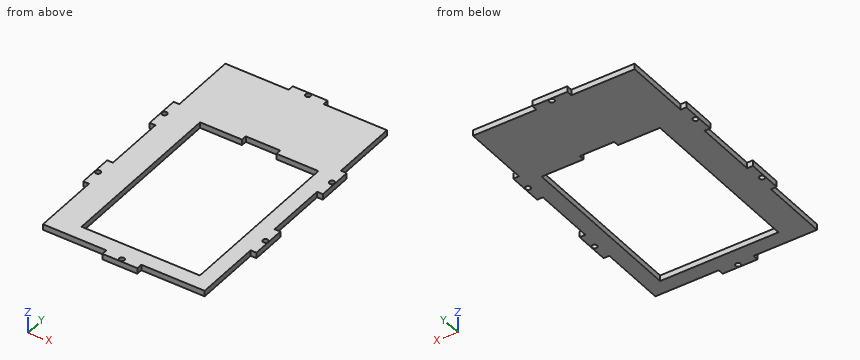
```python
from build123d import *

# Parameters (mm, degrees)
BOSS_EXTRUDE1_DEPTH     = 3.18
CUT_EXTRUDE1_DEPTH      = 87.179315674
SKETCH27_W              = 3.18
SKETCH27_H              = 19.3
BOSS_EXTRUDE9_DEPTH     = 3.18
SKETCH28_W              = 19.3
SKETCH28_H              = 3.18
BOSS_EXTRUDE10_DEPTH    = 3.18
SKETCH29_R              = 1.425
CUT_EXTRUDE14_DEPTH     = 91.550668965
SKETCH30_R              = 1.425
CUT_EXTRUDE15_DEPTH     = 91.550668965
MIRROR9_COPY_1_SKETCH_W = 3.18
MIRROR9_COPY_1_SKETCH_H = 19.3
MIRROR9_COPY_1_DEPTH    = 3.18
MIRROR9_COPY_2_SKETCH_R = 1.425
MIRROR9_COPY_2_DEPTH    = 91.550668965


with BuildPart() as part:
    # Sketch1 → Boss-Extrude1 (new body)
    with BuildSketch(Plane.XY):
        Polygon((-44.645, 73.645), (-14.881666667, 73.645), (14.881666667, 73.645), (44.645, 73.645), (44.645, -73.645), (-44.645, -73.645), align=None)
    extrude(amount=BOSS_EXTRUDE1_DEPTH)

    # Sketch3 → Cut-Extrude1 (cut, through all)
    with BuildSketch(Plane(origin=(0, 0, 0), x_dir=(-1, 0, 0), z_dir=(0, 0, -1))):
        Polygon((-13.10174207, 33.47325793), (-13.10174207, 30.47325793), (-36.27674207, 30.47325793), (-36.27674207, -65.27674207), (29.07325793, -65.27674207), (29.07325793, 30.47325793), (5.89825793, 30.47325793), (5.89825793, 33.47325793), align=None)
    extrude(amount=-CUT_EXTRUDE1_DEPTH, mode=Mode.SUBTRACT)

    # Sketch27 → Boss-Extrude9 (add)
    with BuildSketch(Plane.ZY.offset(44.645)):
        with Locations((1.59, -26.825)):
            Rectangle(SKETCH27_W, SKETCH27_H)
    boss_extrude9 = extrude(amount=BOSS_EXTRUDE9_DEPTH)

    # Sketch28 → Boss-Extrude10 (add)
    with BuildSketch(Plane.XZ.offset(73.645)):
        with Locations((0, 1.59)):
            Rectangle(SKETCH28_W, SKETCH28_H)
    boss_extrude10 = extrude(amount=BOSS_EXTRUDE10_DEPTH)

    # Sketch29 → Cut-Extrude14 (cut, through all)
    with BuildSketch(Plane.XY.offset(3.18)):
        with Locations((-46.235, -26.825)):
            Circle(SKETCH29_R)
    cut_extrude14 = extrude(amount=-CUT_EXTRUDE14_DEPTH, mode=Mode.SUBTRACT)

    # Sketch30 → Cut-Extrude15 (cut, through all)
    with BuildSketch(Plane.XY.offset(3.18)):
        with Locations((0, -75.235)):
            Circle(SKETCH30_R)
    cut_extrude15 = extrude(amount=-CUT_EXTRUDE15_DEPTH, mode=Mode.SUBTRACT)

    # Mirror8: Boss-Extrude9, Cut-Extrude14 across plane
    add(boss_extrude9.mirror(Plane(origin=(0, 0, 0), x_dir=(0, 0, 1), z_dir=(1, 0, 0))))
    add(cut_extrude14.mirror(Plane(origin=(0, 0, 0), x_dir=(0, 0, 1), z_dir=(1, 0, 0))), mode=Mode.SUBTRACT)

    # Mirror9: Boss-Extrude9, Boss-Extrude10, Cut-Extrude14, Cut-Extrude15 across plane
    add(boss_extrude9.mirror(Plane.ZX))
    add(boss_extrude10.mirror(Plane.ZX))
    add(cut_extrude14.mirror(Plane.ZX), mode=Mode.SUBTRACT)
    add(cut_extrude15.mirror(Plane.ZX), mode=Mode.SUBTRACT)

    # Mirror9 copy 1 sketch → Mirror9 copy 1 (add)
    with BuildSketch(Plane(origin=(44.645, 0, 0), x_dir=(0, 0, 1), z_dir=(1, 0, 0))):
        with Locations((1.59, -26.825)):
            Rectangle(MIRROR9_COPY_1_SKETCH_W, MIRROR9_COPY_1_SKETCH_H)
    extrude(amount=MIRROR9_COPY_1_DEPTH)

    # Mirror9 copy 2 sketch → Mirror9 copy 2 (cut, through all)
    with BuildSketch(Plane(origin=(0, 0, 3.18), x_dir=(-1, 0, 0), z_dir=(0, 0, 1))):
        with Locations((-46.235, -26.825)):
            Circle(MIRROR9_COPY_2_SKETCH_R)
    extrude(amount=-MIRROR9_COPY_2_DEPTH, mode=Mode.SUBTRACT)


solid = part.part
```
Geometry check sheet. Reference: the model listing, model coordinates, mm. Round coordinates to 2 decimals unless told otherwise and drop trailing zeros. Order: outer loops, then holes, each group sorted by start corner. A loop starts at its lowest first (then second) coordinate and runs counter-clockwise, first axis right, second up. Notation, with made-up numbers: (62.5, 19.25) - (110.5, 19.25) arc R37 ccw to (110.5, 57.25) - close; hole circle Ø10 at (21, 55). An arc over 180 degrees is marked (long way). Use a Markdown table: item, result. Add a question column.
(1) Sectioned sample at B-B, the plane x = 30.5. Enter the section's corners in (y, z) (3 decimals), and give its area (3 significant figures).
(2) Sectioned sample at D-D, the plane z = 0.7. Count the separate pieces of the cut face and the enclosed holes in it, and give its area (3 significant figures).
(3) Material ranges on line 1 along Y through (x, z) = (0, 0.9) (3 decimals); line 2 along X through (y, z) = (-58, 2.75) (3 decimals); line 3 along Y through (x, z) = (9, 3.05) (3 decimals), recorded low to high. Write a range as [from, to].
(4) Sectioned sample at C-C, the plane x = -35.5. Enter the section's corners in (y, z) (3 decimals), and give its area (3 significant figures).
(5) Depth check by flat-ended pin: pin 1 (1 mm diameter, centred on y = 76, z = 1, fed in from +X); pin 2 (1 mm diameter, centred on x = 46.5, z = 2.5, fed in from -Y) (3 decimals); pin 3 (1.6 mm diameter, centred on y = -11.5, z = 1.5, fed in from +X) (3 decimals). Enter the tip coordinate at first touch or a pass-through.
(6) Sectioned sample at A-A, the plane y = -15. Enter the section's corners in (x, z) (3 decimals).
Answers below:
| question | item | result |
|---|---|---|
| 1 | outline | (-73.645, 0) - (-65.277, 0) - (-65.277, 3.18) - (-73.645, 3.18) - close; (30.473, 0) - (73.645, 0) - (73.645, 3.18) - (30.473, 3.18) - close |
| 1 | area | 164 mm² |
| 2 | separate pieces | 1 |
| 2 | enclosed holes | 7 |
| 2 | area | 7,170 mm² |
| 3 | line 1 | [-76.825, -76.66], [-73.81, -65.277], [33.473, 73.81], [76.66, 76.825] |
| 3 | line 2 | [-44.645, -29.073], [36.277, 44.645] |
| 3 | line 3 | [-76.825, -65.277], [33.473, 76.825] |
| 4 | outline | (-73.645, 0) - (73.645, 0) - (73.645, 3.18) - (-73.645, 3.18) - close |
| 4 | area | 468 mm² |
| 5 | pin 1 | x = 9.65 |
| 5 | pin 2 | y = -36.475 |
| 5 | pin 3 | x = 44.645 |
| 6 | outline | (-44.645, 0) - (-29.073, 0) - (-29.073, 3.18) - (-44.645, 3.18) - close; (36.277, 0) - (44.645, 0) - (44.645, 3.18) - (36.277, 3.18) - close |
